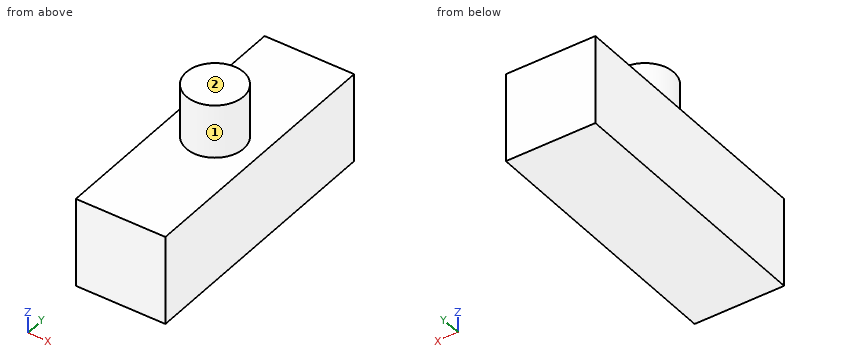
from build123d import *

# Parameters (mm, degrees)
F1_R     = 12.209968
F2_DEPTH = 41.91
F0_W     = 114.3
F0_H     = 38.1
F3_DEPTH = 19.05


with BuildPart() as f2:
    # F1 (on Top) → F2 (new body)
    with BuildSketch(Plane.XY):
        Circle(F1_R)
    extrude(amount=F2_DEPTH)

    # F0 (on Right) → F3 (join, symmetric)
    with BuildSketch(Plane.YZ):
        Rectangle(F0_W, F0_H)
    extrude(amount=F3_DEPTH, both=True)


solid = f2.part
Geometry: final body of the model. Coordinates: model frame, mm. Face numbers are marked on the shaded views. A direction names the side the tool comes from. Give positions to 0.01 mm unless a question says otherwise; leave off trailing zeros. Loops run counter-clockwise (first coordinate to the right, second up) from the corner with the lowest first, then second, coordinate; pieces in that order, holes last. Notation, with made-up numbers: (3.5, 25.25) -> (49.5, 25.25) arc R27 cw to (49.5, 44.25) -> close; hole circle Ø3 at (80, 23.5). An arc over 180 degrees is marked (long way). Put each result on its own line as item: value.
1. Cut plane B-B (y = 0). Return the cut outline in (x, z).
Taken from the geometry:
outline: (-19.05, -19.05) -> (19.05, -19.05) -> (19.05, 19.05) -> (12.21, 19.05) -> (12.21, 41.91) -> (-12.21, 41.91) -> (-12.21, 19.05) -> (-19.05, 19.05) -> close
2. Cut plane D-D (x = -14). Return the cut outline in (y, z), plus the area to 3 significant figures.
Taken from the geometry:
outline: (-57.15, -19.05) -> (57.15, -19.05) -> (57.15, 19.05) -> (-57.15, 19.05) -> close
area: 4,350 mm2
3. Ray query, line 1 along Z through (x, y) = (-6, -14); line 2 along Y through (x, z) = (-11, 26.5); line 3 along Y through (x, z) = (6.5, 23.5). Return the intervals inside material, ascending. Write a range as [from, to].
Taken from the geometry:
line 1: z = [-19.05, 19.05]
line 2: y = [-5.3, 5.3]
line 3: y = [-10.34, 10.34]
4. Pin query (flat end, axial travel): P1, Ø3, axis at x = 12, z = 25, coming from the -Y side; P2, Ø1, axis at x = -4.5, z = 23.5, coming from the +Y side; P3, Ø1.5, axis at x = 11.5, z = 23.5, coming from the -Y side. Return the tip coordinate at first contact, or that it passes through.
Taken from the geometry:
P1: stops at y = -6.23
P2: stops at y = 11.54
P3: stops at y = -5.79
5. Cut plane C-C (z = 25). Return the cut outline in (x, y).
Taken from the geometry:
outline: circle Ø24.42 at (0, 0)
6. Cut plane A-A (x = 0). Return the cut outline in (y, z).
Taken from the geometry:
outline: (-57.15, -19.05) -> (57.15, -19.05) -> (57.15, 19.05) -> (12.21, 19.05) -> (12.21, 41.91) -> (-12.21, 41.91) -> (-12.21, 19.05) -> (-57.15, 19.05) -> close
7. Set-up query: the marked faces 1 and 2. Return all of +Z, -Z, +X, -X, +Y, -Y with unobstructed straight access to the full face (end or side cutting, diameter ignored); none if empty.
Taken from the geometry:
face 1: +Z
face 2: +Z, +X, -X, +Y, -Y
